```python
from build123d import *

# Parameters (mm, degrees)
F0_W      = 4.55
F0_H      = 4.6
F0_W_2    = 10.6
F0_H_2    = 0.55
F1_DEPTH  = 0.4
F2_R      = 1.2
F3_DEPTH  = 0.5
F4_R      = 0.39999
F5_W      = 10.6
F5_H      = 5.7
F6_DEPTH  = 5.2
F7_R      = 1
F8_W      = 6.2
F8_H      = 3.4
F9_DEPTH  = 0.4
F10_W     = 3
F10_H     = 3
F11_DEPTH = 5.6
F12_W     = 7.6
F12_H     = 0.4
F13_DEPTH = 2.2


# Not quite as in the source:
# - a fillet or chamfer is up to 0.001 mm smaller than in the source, because OpenCascade refuses the exact size


with BuildPart() as f1:
    # F0 (on Front) → F1 (new body)
    with BuildSketch(Plane.XZ):
        with Locations((7.575, 0)):
            Rectangle(F0_W, F0_H)
        with Locations((0, -2.575)):
            Rectangle(F0_W_2, F0_H_2)
        Rectangle(F0_W_2, F0_H)
        with Locations((-7.575, 0)):
            Rectangle(F0_W, F0_H)
        with Locations((0, 2.575)):
            Rectangle(F0_W_2, F0_H_2)
    extrude(amount=F1_DEPTH)

    # F2 (on face) → F3 (cut)
    with BuildSketch(Plane.XZ.offset(0.4)):
        with Locations((-7.35, 0)):
            Circle(F2_R)
        with Locations((7.35, 0)):
            Circle(F2_R)
    extrude(amount=-F3_DEPTH, mode=Mode.SUBTRACT)

    # F4 (radius 0.4 in the source; OpenCascade refuses exactly that, so slightly less here)
    f4_edges = [f1.edges().sort_by_distance(p)[0] for p in [
        (0, -0.4, 2.85),
        (0, -0.4, -2.85),
    ]]
    fillet(f4_edges, radius=F4_R)

    # F5 (on face) → F6 (join)
    with BuildSketch(Plane(origin=(0, 0, 0), x_dir=(-1, 0, 0), z_dir=(0, 1, 0))):
        Rectangle(F5_W, F5_H)
    extrude(amount=F6_DEPTH)

    # F7
    f7_edges = [f1.edges().sort_by_distance(p)[0] for p in [
        (9.85, -0.2, 2.3),
        (9.85, -0.2, -2.3),
        (-9.85, -0.2, -2.3),
        (-9.85, -0.2, 2.3),
    ]]
    fillet(f7_edges, radius=F7_R)

    # F8 (on face) → F9 (cut)
    with BuildSketch(Plane.XZ.offset(0.4)):
        Rectangle(F8_W, F8_H)
    extrude(amount=-F9_DEPTH, mode=Mode.SUBTRACT)

    # F10 (on face) → F11 (join)
    with BuildSketch(Plane.XZ):
        with Locations((-1.6, 0)):
            Rectangle(F10_W, F10_H)
    extrude(amount=F11_DEPTH)

    # F12 (on face) → F13 (join)
    with BuildSketch(Plane(origin=(0, 5.2, 0), x_dir=(-1, 0, 0), z_dir=(0, 1, 0))):
        Rectangle(F12_W, F12_H)
    extrude(amount=F13_DEPTH)


solid = f1.part
```
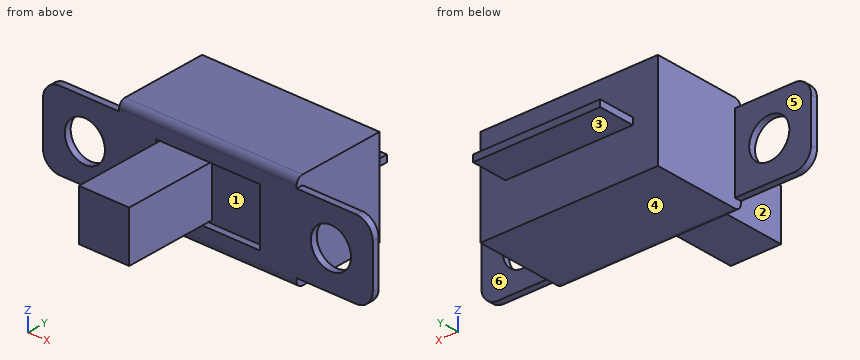
Geometry check sheet. Reference: the model listing, model coordinates, mm. Face numbers are marked on the shaded views. A direction names the side the tool comes from. Give positions to 0.01 mm unless a question says otherwise; leave off trailing zeros. Write each loop counter-clockwise with the first axis right and the second up, starting at its lowest first coordinate (ties: lowest second). Pieces come first, ordered by that corner, then holes. Notation, with made-up numbers: (27.25, -9.75) - (63.25, -9.75) arc R13 ccw to (63.25, -0.75) - close; hole circle Ø11 at (-11.5, -36.5). An arc over 180 degrees is marked (long way). Use a Markdown table: item, result.
Q1. Set-up check for the marked faces 4, 5 and 6: record each of +Z, -Z, +X, -X, +Y, -Y from which the full face is reachable in a straight line by a thin tool's end or side.
Computed:
| item | result |
|---|---|
| face 4 | -Z, +X, -X, +Y, -Y |
| face 5 | +Z, -Z, -X, +Y |
| face 6 | +Z, -Z, +X, +Y |
Q2. Section check C-C, the plane x = -2.25. Enter the section's corners in (y, z).
Computed:
| item | result |
|---|---|
| outline | (-5.6, -1.5) - (0, -1.5) - (0, -1.7) - (-0.4, -1.7) - (-0.4, -2.45) arc R0.4 ccw to (0, -2.85) - (5.2, -2.85) - (5.2, -0.2) - (7.4, -0.2) - (7.4, 0.2) - (5.2, 0.2) - (5.2, 2.85) - (0, 2.85) arc R0.4 ccw to (-0.4, 2.45) - (-0.4, 1.7) - (0, 1.7) - (0, 1.5) - (-5.6, 1.5) - close |
Q3. Draft check along X on the marked faces 1, 2 and 3. Enter one of: pulls with the +X half, pulls with the -X half, needs draft (parallel to the pull), parting line crosses it, or undercut.
Computed:
| item | result |
|---|---|
| face 1 | undercut |
| face 2 | pulls with the -X half |
| face 3 | needs draft |
Q4. Thickness scan on L1, parallel to Z at x = -7.35, y = -0.2; L2, parallel to Y at x = 6.25, z = 1.4; L3, parallel to Y at x = 2.5, z = -1.6. Record the ranges inside material, lowest first. Write a range as [from, to].
Computed:
| item | result |
|---|---|
| L1 | z = [-2.3, -1.2], [1.2, 2.3] |
| L2 | y = [-0.4, 0] |
| L3 | y = [0, 5.2] |
Q5. Section check A-A, the plane z = 0. Enter the section's corners in (x, y).
Computed:
| item | result |
|---|---|
| outline | (-9.85, -0.4) - (-8.55, -0.4) - (-8.55, 0) - (-9.85, 0) - close; (-6.15, -0.4) - (-3.1, -0.4) - (-3.1, -5.6) - (-0.1, -5.6) - (-0.1, 0) - (3.1, 0) - (3.1, -0.4) - (6.15, -0.4) - (6.15, 0) - (5.3, 0) - (5.3, 5.2) - (3.8, 5.2) - (3.8, 7.4) - (-3.8, 7.4) - (-3.8, 5.2) - (-5.3, 5.2) - (-5.3, 0) - (-6.15, 0) - close; (8.55, -0.4) - (9.85, -0.4) - (9.85, 0) - (8.55, 0) - close |
Q6. Section check D-D, the plane y = 2.25. Enter the section's corners in (x, z), then the cut area to 3 significant figures.
Computed:
| item | result |
|---|---|
| outline | (-5.3, -2.85) - (5.3, -2.85) - (5.3, 2.85) - (-5.3, 2.85) - close |
| area | 60.4 mm² |
Q7. Go/stop test with flat-tipped pins: P1, Ø1.7, axis at x = 1.5, z = -0.5, coming from the +Y side; P2, Ø3, axis at y = 2, z = 1, coming from the +X side; P3, Ø1.4, axis at x = -7, z = -0.5, coming from the +Y side; P4, Ø1.4, axis at x = -7.35, z = 0, coming from the +Y side. Record where each tip stops, or that it passes through.
Computed:
| item | result |
|---|---|
| P1 | stops at y = 7.4 |
| P2 | stops at x = 5.3 |
| P3 | stops at y = 0 |
| P4 | passes through |
Q8. Section check B-B, the plane x = -7.35. Enter the section's corners in (y, z), then the cut area to 3 significant figures.
Computed:
| item | result |
|---|---|
| outline | (-0.4, -2.3) - (0, -2.3) - (0, -1.2) - (-0.4, -1.2) - close; (-0.4, 1.2) - (0, 1.2) - (0, 2.3) - (-0.4, 2.3) - close |
| area | 0.880 mm² |
